Build history of the part. All positions in model axes, mm. Give positions to 0.01 mm unless a question says otherwise; leave off trailing zeros. Loops run counter-clockwise (first coordinate to the right, second up) from the corner with the lowest first, then second, coordinate; pieces in that order, holes last.
1) Band-saw the part on A-A on y = 12. List the corners of the cut face in (x, z), then the cut area to 3 significant figures.
2) Band-saw the part on B-B on x = 1.5. List the corners of the cut face in (y, z).
3) Band-saw the part on C-C on z = -2.5. List the corners of the cut face in (x, y), then the cut area to 3 significant figures.
4) Band-saw the part on D-D on x = -12.5. List the corners of the cut face in (y, z), then the cut area to 3 significant figures.
5) Flat gauge pins, fed straight in: P1, Ø2, axis at x = -9, z = -0.5, coming from the +Y side; P2, Ø1.5, axis at y = 9, z = -2.5, coming from the +X side; P3, Ø17, axis at x = 0, y = 0, coming from the +Z side. Where does each tip first touch, or does it go through?
6) Wall check: line 1 (X direction, y = 0, z = -2.85); line 2 (Y direction, x = 0, z = -2.4); line 3 (X direction, y = 9, z = -1.85). Give the ranges that are in metal, low to high.
```python
from build123d import *

# Parameters (mm, degrees)
SKETCH_1_W          = 16.02
SKETCH_1_H          = 4
CUT_EXTRUDE_1_DEPTH = 24.006103538
DRAFT_1_ANGLE       = -30
DRAFT_2_ANGLE       = 30
SKETCH_3_W          = 10.52
SKETCH_3_H          = 4


with BuildPart() as part:
    # 草图1 → 旋转1 (revolve)
    with BuildSketch(Plane(origin=(0, 0, 0), x_dir=(1, 0, 0), z_dir=(0, 1, 0))):
        with Locations((8.01, 2)):
            Rectangle(SKETCH_1_W, SKETCH_1_H)
    revolve(axis=Axis((0, 0, -4), (0, 0, 1)))

    # 草图2 → 切除-拉伸1 (cut, through all)
    with BuildSketch(Plane.XY):
        with BuildLine():
            Line((0, 16.02), (0, 10.52))
            ThreePointArc((0, 10.52), (1.16180729, 10.455649373), (2.309401077, 10.263384757))
            Line((2.309401077, 10.263384757), (2.309401077, 15.852667494))
            ThreePointArc((2.309401077, 15.852667494), (1.157727677, 15.978112111), (0, 16.02))
        make_face()
    extrude(amount=-CUT_EXTRUDE_1_DEPTH, mode=Mode.SUBTRACT)

    # 拔模1
    draft_1_faces = [part.faces().sort_by_distance(p)[0] for p in [
        (0, 13.27, -2),
    ]]
    draft(draft_1_faces, Plane.XY, DRAFT_1_ANGLE)

    # 拔模2
    draft_2_faces = [part.faces().sort_by_distance(p)[0] for p in [
        (2.309401077, 13.058026125, -2),
    ]]
    draft(draft_2_faces, Plane.XY, DRAFT_2_ANGLE)

    # 草图3 → 切除-旋转1 (revolve, cut)
    with BuildSketch(Plane.XZ):
        with Locations((5.26, -2)):
            Rectangle(SKETCH_3_W, SKETCH_3_H)
    revolve(axis=Axis((0, 0, 0), (0, 0, -1)), mode=Mode.SUBTRACT)


solid = part.part
```
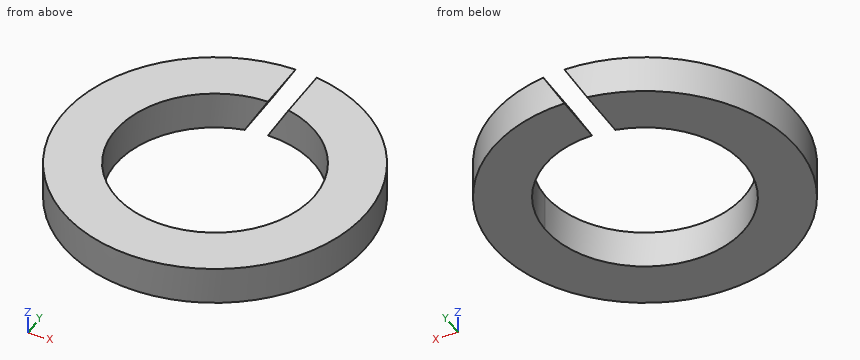
Findings below:
1. outline: (-10.61, -4) - (-2.31, -4) - (0, 0) - (-10.61, 0) - close; (0, -4) - (10.61, -4) - (10.61, 0) - (2.31, 0) - close
1. area: 75.7 mm2
2. outline: (-15.95, -4) - (-10.41, -4) - (-10.41, 0) - (-15.95, 0) - close; (10.41, -4) - (15.95, -4) - (15.95, -1.4) - (10.41, -1.4) - close
3. outline: (-1.44, 10.42) - (-1.44, 15.95) arc R16.02 ccw (long way) to (0.87, 16) - (0.87, 10.48) arc R10.52 cw (long way) to start
3. area: 446 mm2
4. outline: (-10.02, -4) - (10.02, -4) - (10.02, 0) - (-10.02, 0) - close
4. area: 80.2 mm2
5. P1: stops at y = 13.88
5. P2: stops at x = 13.73
5. P3: passes through
6. line 1: x = -16.02 to -10.52, 10.52 to 16.02
6. line 2: y = -16.02 to -10.52
6. line 3: x = -13.25 to -5.45, 5.45 to 13.25
